Autodesk Inventor part; units mm, degrees
ref_plane "Plano inicial" through (0, 0, 0) normal (0, 0, 1) x (1, 0, 0)
ref_plane "Plano final" through (0, 0, 648.3012) normal (0, 0, 1) x (1, 0, 0)
ref_plane "Plano de trabajo4" through (0, 20, 650) normal (0, -0.7071, 0.7071) x (1, 0, 0)
ref_plane "Plano inicial" through (0, 0, 0) normal (0, 0, 1) x (1, 0, 0)
ref_plane "Plano final" through (0, 0, 648.3012) normal (0, 0, 1) x (1, 0, 0)
sketch "Boceto" plane through (0, 0, 0) normal (0, 0, 1) x (1, 0, 0)
  line L0 (-14.2, 20) -> (14.2, 20)
  line L1 (20, 14.2) -> (20, -14.2)
  line L2 (14.2, -20) -> (-14.2, -20)
  line L3 (-20, -14.2) -> (-20, 14.2)
  arc A0 (-14.2, 20) -> (-20, 14.2) centre (-14.2, 14.2) ccw
  arc A1 (20, 14.2) -> (14.2, 20) centre (14.2, 14.2) ccw
  arc A2 (14.2, -20) -> (20, -14.2) centre (14.2, -14.2) ccw
  arc A3 (-20, -14.2) -> (-14.2, -20) centre (-14.2, -14.2) ccw
  line L4 (-29.6817, 0) -> (29.6817, 0) construction
  line L5 (0, -29.6817) -> (0, 29.6817) construction
  arc A4 (-14.2, 17.1) -> (-17.1, 14.2) centre (-14.2, 14.2) ccw
  line L6 (-14.2, 17.1) -> (14.2, 17.1)
  arc A5 (17.1, 14.2) -> (14.2, 17.1) centre (14.2, 14.2) ccw
  line L7 (17.1, 14.2) -> (17.1, -14.2)
  arc A6 (14.2, -17.1) -> (17.1, -14.2) centre (14.2, -14.2) ccw
  line L8 (14.2, -17.1) -> (-14.2, -17.1)
  arc A7 (-17.1, -14.2) -> (-14.2, -17.1) centre (-14.2, -14.2) ccw
  line L9 (-17.1, -14.2) -> (-17.1, 14.2)
  point P0 (-20, 20)
  point P1 (20, -20)
  point P2 (20, 20)
  dimension "b" = 40
  dimension "msp_r" = 5.8
  dimension "d8" = 20
  dimension "d9" = 20
  dimension "d10" = 2.9
extrude "Cuerpo" add sketch "Boceto" along normal up to surface (648.3012 mm away) from surface at 0
sketch "Sketch2" plane through (0, 0, 0) normal (0, 0, 1) x (1, 0, 0)
  line L0 (0, 0) -> (10, 0)
ref_plane "Work Plane3" through (0, 0, 0) normal (0, -1, 0) x (1, 0, 0)
sketch "Sketch3" plane through (0, 0, 0) normal (0, -1, 0) x (1, 0, 0)
  line L0 (-2, 0) -> (12, 0)
  line L1 (-2, 648.3012) -> (12, 648.3012)
  dimension "d14" = 648.3012
ref_plane "Plano de trabajo4" through (0, 20, 650) normal (0, -0.7071, 0.7071) x (1, 0, 0)
split "Dividir1" plane through (0, 20, 650) removes the side toward (0, -0.7071, 0.7071)
ref_plane "Plano de trabajo5" through (-20, 0, 650) normal (0.7071, 0, 0.7071) x (0.7071, 0, -0.7071)
split "Dividir2" plane through (-20, 0, 650) removes the side toward (0.7071, 0, 0.7071)
equation "\"msp_r\" = 2 * ParT"
equation "\"d8\" = d9"
equation "\"d9\" = 0.5 * b"
equation "\"d10\" = ParT"
equation "\"G_OFFSET_START\" = 0"
equation "\"G_OFFSET_END\" = 18.30122"
equation "\"d12\" = G_OFFSET_END + B_L"
equation "\"G_L\" = d14"
properties part number "DIN 59 410 - 40x40x2.9-648.301" material "Acero, suave"
Work out the finished part from the listing and answer in its coordinate system (mm). A direction names the side the tool comes from. Give positions to 0.01 mm unless a question says otherwise; leave off trailing zeros. Write each loop counter-clockwise with the first axis right and the second up, starting at its lowest first coordinate (ties: lowest second). Pieces come first, ordered by that corner, then holes.
Q1. The part is cut by section C-C on z = 291. Give the vertices of the cut face in (x, y).
Answer:
outline: (-20, -14.2) arc R5.8 ccw to (-14.2, -20) - (14.2, -20) arc R5.8 ccw to (20, -14.2) - (20, 14.2) arc R5.8 ccw to (14.2, 20) - (-14.2, 20) arc R5.8 ccw to (-20, 14.2) - close; hole (-17.1, -14.2) arc R2.9 ccw to (-14.2, -17.1) - (14.2, -17.1) arc R2.9 ccw to (17.1, -14.2) - (17.1, 14.2) arc R2.9 ccw to (14.2, 17.1) - (-14.2, 17.1) arc R2.9 ccw to (-17.1, 14.2) - close
Q2. The part is cut by section B-B on y = -6. Give the vertices of the cut face in (x, z).
Answer:
outline: (-20, 0) - (-17.1, 0) - (-17.1, 624) - (-20, 624) - close; (17.1, 0) - (20, 0) - (20, 610) - (17.1, 612.9) - close
Q3. Straight lines are drawn through the part: L1, parallel to Y at x = -10.5, z = 459; L2, parallel to X at y = 15, z = 206.5. For each, find the intervals that lie inside material, in ascending order.
Answer:
L1: y = -20 to -17.1, 17.1 to 20
L2: x = -19.94 to -16.99, 16.99 to 19.94
Q4. The part is cut by section A-A on x = -7. Give the vertices of the cut face in (y, z), and give its area (3 significant figures).
Answer:
outline: (-20, 0) - (-17.1, 0) - (-17.1, 612.9) - (-20, 610) - close; (17.1, 0) - (20, 0) - (20, 637) - (17.1, 637) - close
area: 3,620 mm2
Q5. A tool of negligible diameter and unlimited length cuts with its end or side. For faces 4 (the face through (0, 17.1, 318)), 5 (the face through (-18, 0, 0)), from which of +Z, -Z, +X, -X, +Y, -Y can it reach the whole face along a straight path? Write none if from no direction.
Answer:
face 4: +Z, -Z
face 5: -Z, +X, -X, +Y, -Y
Q6. For a pull along X with two mould halves and no side action, classify faces 1 (the face through (0, -20, 301)), 2 (the face through (-17.1, 0, 318)), 3 (the face through (20, 0, 301)) as released by +X, released by -X, zero draft, split by the parting line, or undercut.
Answer:
face 1: zero draft
face 2: undercut
face 3: released by +X
